Input: dimensioned drawing with shaded views. Units: mm. Origin: part minimum x, y, z. A direction names the side the tool comes from. Coordinates: 2 decimals unless noted, no trailing zeros. Order: outer loops, then holes, each group sorted by start corner. A loop starts at its lowest first (then second) coordinate and runs counter-clockwise, first axis right, second up. Notation, with made-up numbers: M 25,78 L 67,78 A14 ccw 67,99 Z; hole C 17,35.25 d5. An arc over 180 degrees is marked long. Write item = value, one per line.
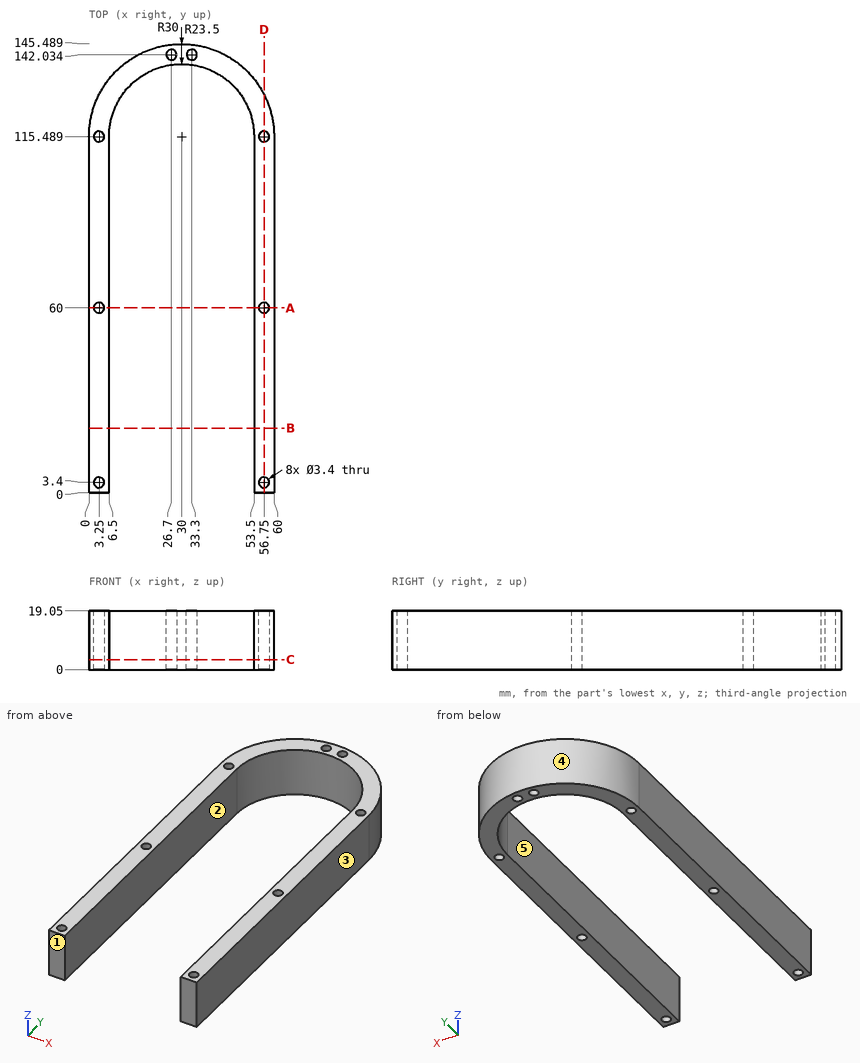
1) Section C-C, the plane z = 3.25. Give the number of separate pieces and of enclosed holes in the cut face.
Numbers:
separate_pieces = 1
enclosed_holes = 8
2) Section B-B, the plane y = 21. Return loops of the section in (x, z).
Numbers:
outline = M 0,0 L 6.5,0 L 6.5,19.05 L 0,19.05 Z; M 53.5,0 L 60,0 L 60,19.05 L 53.5,19.05 Z
3) Mould query, pull axis X, two halves, no side actions, for the marked faces 1, 2 and 3. Classes: pulls with the +X half, pulls with the -X half, needs draft (parallel to the pull), parting line crosses it, or undercut.
Numbers:
face_1 = needs draft
face_2 = undercut
face_3 = pulls with the +X half
4) Pin query (flat end, axial travel): pin 1 (4 mm diameter, centred on x = 38.5, z = 10, fed in from +Y); pin 2 (6 mm diameter, centred on x = 44, z = 9.5, fed in from +Y); pin 3 (10 mm diameter, centred on x = 52.5, z = 13.5, fed in from -Y); pin 4 (1 mm diameter, centred on x = 21.5, z = 9, fed in from +Y). Return the tip coordinate at first contact, or that it passes through.
Numbers:
pin_1 = 144.78
pin_2 = 143.4
pin_3 = 0
pin_4 = 144.4
5) Set-up query: the marked faces 4 and 5. Return all of +Z, -Z, +X, -X, +Y, -Y with unobstructed straight access to the full face (end or side cutting, diameter ignored); none if empty.
Numbers:
face_4 = +Z, -Z, +Y
face_5 = +Z, -Z, -Y
6) Line query: L1, parallel to X at y = 60, z = 7.5; L2, parallel to X at y = 55, z = 4.5; L3, parallel to Y at x = 3.25, z = 12.5 (1 decimal). Output: solid intervals per line, ascending.
Numbers:
L1 = 0 to 1.55, 4.95 to 6.5, 53.5 to 55.05, 58.45 to 60
L2 = 0 to 6.5, 53.5 to 60
L3 = 0 to 1.7, 5.1 to 58.3, 61.7 to 113.8, 117.2 to 129.1
7) Section D-D, the plane x = 56.75. Return loops of the section in (y, z).
Numbers:
outline = M 0,0 L 1.7,0 L 1.7,19.05 L 0,19.05 Z; M 5.1,0 L 58.3,0 L 58.3,19.05 L 5.1,19.05 Z; M 61.7,0 L 113.79,0 L 113.79,19.05 L 61.7,19.05 Z; M 117.19,0 L 129.07,0 L 129.07,19.05 L 117.19,19.05 Z
8) Section A-A, the plane y = 60. Return loops of the section in (x, z).
Numbers:
outline = M 0,0 L 1.55,0 L 1.55,19.05 L 0,19.05 Z; M 4.95,0 L 6.5,0 L 6.5,19.05 L 4.95,19.05 Z; M 53.5,0 L 55.05,0 L 55.05,19.05 L 53.5,19.05 Z; M 58.45,0 L 60,0 L 60,19.05 L 58.45,19.05 Z
